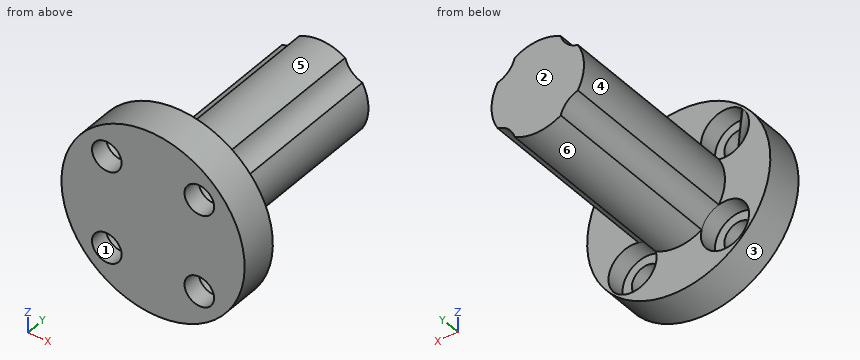
```python
from build123d import *
from build123d.topology import SkipClean

# Parameters (mm, degrees)
SKETCH1_R           = 9.9
BOSS_EXTRUDE1_DEPTH = 4
SKETCH2_R           = 5
BOSS_EXTRUDE2_DEPTH = 20
CUT_EXTRUDE1_REACH  = 26.414
SKETCH3_R           = 1.6
CUT_EXTRUDE2_REACH  = 26.414
SKETCH3_3_R         = 2.6
SKETCH3_3_R_2       = 1.6
SKETCH3_4_R         = 2.6
SKETCH3_4_R_2       = 1.6
CUT_EXTRUDE3_DEPTH  = 2


with BuildPart() as part:
    # Sketch1 → Boss-Extrude1 (new body)
    with BuildSketch(Plane(origin=(0, 0, 0), x_dir=(1, 0, 0), z_dir=(0, 1, 0))):
        with Locations(Location((0, 0, 0), (0, 0, 270))):
            Circle(SKETCH1_R)
    extrude(amount=BOSS_EXTRUDE1_DEPTH)

    # Sketch2 → Boss-Extrude2 (add)
    with BuildSketch(Plane(origin=(0, 4, 0), x_dir=(1, 0, 0), z_dir=(0, 1, 0))):
        with Locations(Location((0, 0, 0), (0, 0, 270))):
            Circle(SKETCH2_R)
    extrude(amount=BOSS_EXTRUDE2_DEPTH)

    # Sketch3 → Cut-Extrude1 (cut, up to next)
    with BuildSketch(Plane(origin=(0, 4, 0), x_dir=(1, 0, 0), z_dir=(0, 1, 0)), mode=Mode.PRIVATE) as cut_extrude1_sk1:
        with Locations(Location((5, 5, 0), (0, 0, 270))):
            Circle(SKETCH3_R)
    cut_extrude1_tool1 = extrude(cut_extrude1_sk1.sketch, amount=-CUT_EXTRUDE1_REACH, mode=Mode.PRIVATE) & part.part
    # Sketch3 → Cut-Extrude1 (cut, up to next)
    with BuildSketch(Plane(origin=(0, 4, 0), x_dir=(1, 0, 0), z_dir=(0, 1, 0)), mode=Mode.PRIVATE) as cut_extrude1_sk2:
        with Locations(Location((5, -5, 0), (0, 0, 270))):
            Circle(SKETCH3_R)
    cut_extrude1_tool2 = extrude(cut_extrude1_sk2.sketch, amount=-CUT_EXTRUDE1_REACH, mode=Mode.PRIVATE) & part.part
    # Sketch3 → Cut-Extrude1 (cut, up to next)
    with BuildSketch(Plane(origin=(0, 4, 0), x_dir=(1, 0, 0), z_dir=(0, 1, 0)), mode=Mode.PRIVATE) as cut_extrude1_sk3:
        with Locations(Location((-5, -5, 0), (0, 0, 270))):
            Circle(SKETCH3_R)
    cut_extrude1_tool3 = extrude(cut_extrude1_sk3.sketch, amount=-CUT_EXTRUDE1_REACH, mode=Mode.PRIVATE) & part.part
    # Sketch3 → Cut-Extrude1 (cut, up to next)
    with BuildSketch(Plane(origin=(0, 4, 0), x_dir=(1, 0, 0), z_dir=(0, 1, 0)), mode=Mode.PRIVATE) as cut_extrude1_sk4:
        with Locations(Location((-5, 5, 0), (0, 0, 270))):
            Circle(SKETCH3_R)
    cut_extrude1_tool4 = extrude(cut_extrude1_sk4.sketch, amount=-CUT_EXTRUDE1_REACH, mode=Mode.PRIVATE) & part.part
    add(cut_extrude1_tool1.solids().sort_by_distance((5, 4, -5))[0], mode=Mode.SUBTRACT)
    add(cut_extrude1_tool2.solids().sort_by_distance((5, 4, 5))[0], mode=Mode.SUBTRACT)
    add(cut_extrude1_tool3.solids().sort_by_distance((-5, 4, 5))[0], mode=Mode.SUBTRACT)
    add(cut_extrude1_tool4.solids().sort_by_distance((-5, 4, -5))[0], mode=Mode.SUBTRACT)

    # Sketch3_3 → Cut-Extrude2 (cut, up to next)
    with BuildSketch(Plane(origin=(0, 4, 0), x_dir=(1, 0, 0), z_dir=(0, 1, 0)), mode=Mode.PRIVATE) as cut_extrude2_sk1:
        with Locations((5, 5)):
            Circle(SKETCH3_3_R)
        with Locations(Location((5, 5, 0), (0, 0, 270))):
            Circle(SKETCH3_3_R_2, mode=Mode.SUBTRACT)
    cut_extrude2_tool1 = extrude(cut_extrude2_sk1.sketch, amount=CUT_EXTRUDE2_REACH, mode=Mode.PRIVATE) & part.part
    # Sketch3_3 → Cut-Extrude2 (cut, up to next)
    with BuildSketch(Plane(origin=(0, 4, 0), x_dir=(1, 0, 0), z_dir=(0, 1, 0)), mode=Mode.PRIVATE) as cut_extrude2_sk2:
        with Locations((-5, 5)):
            Circle(SKETCH3_3_R)
        with Locations(Location((-5, 5, 0), (0, 0, 270))):
            Circle(SKETCH3_3_R_2, mode=Mode.SUBTRACT)
    cut_extrude2_tool2 = extrude(cut_extrude2_sk2.sketch, amount=CUT_EXTRUDE2_REACH, mode=Mode.PRIVATE) & part.part
    # Sketch3_3 → Cut-Extrude2 (cut, up to next)
    with BuildSketch(Plane(origin=(0, 4, 0), x_dir=(1, 0, 0), z_dir=(0, 1, 0)), mode=Mode.PRIVATE) as cut_extrude2_sk3:
        with Locations((-5, -5)):
            Circle(SKETCH3_3_R)
        with Locations(Location((-5, -5, 0), (0, 0, 270))):
            Circle(SKETCH3_3_R_2, mode=Mode.SUBTRACT)
    cut_extrude2_tool3 = extrude(cut_extrude2_sk3.sketch, amount=CUT_EXTRUDE2_REACH, mode=Mode.PRIVATE) & part.part
    # Sketch3_3 → Cut-Extrude2 (cut, up to next)
    with BuildSketch(Plane(origin=(0, 4, 0), x_dir=(1, 0, 0), z_dir=(0, 1, 0)), mode=Mode.PRIVATE) as cut_extrude2_sk4:
        with Locations((5, -5)):
            Circle(SKETCH3_3_R)
        with Locations(Location((5, -5, 0), (0, 0, 270))):
            Circle(SKETCH3_3_R_2, mode=Mode.SUBTRACT)
    cut_extrude2_tool4 = extrude(cut_extrude2_sk4.sketch, amount=CUT_EXTRUDE2_REACH, mode=Mode.PRIVATE) & part.part
    add(cut_extrude2_tool1.solids().sort_by_distance((2.473539, 4, -5))[0], mode=Mode.SUBTRACT)
    add(cut_extrude2_tool2.solids().sort_by_distance((-7.526461, 4, -5))[0], mode=Mode.SUBTRACT)
    add(cut_extrude2_tool3.solids().sort_by_distance((-7.526461, 4, 5))[0], mode=Mode.SUBTRACT)
    add(cut_extrude2_tool4.solids().sort_by_distance((2.473539, 4, 5))[0], mode=Mode.SUBTRACT)

    # Sketch3_4 → Cut-Extrude3 (cut)
    # profile 1 of 4: a face of its own
    with SkipClean():  # the faces are left unmerged after this step: merging them gives an invalid solid
        with BuildSketch(Plane(origin=(0, 4, 0), x_dir=(1, 0, 0), z_dir=(0, 1, 0))):
            with Locations(Location((5, 5, 0), (0, 0, 194.741200994))):
                Circle(SKETCH3_4_R)
            with Locations(Location((5, 5, 0), (0, 0, 270))):
                Circle(SKETCH3_4_R_2, mode=Mode.SUBTRACT)
        # profile 2 of 4: a face of its own
        with BuildSketch(Plane(origin=(0, 4, 0), x_dir=(1, 0, 0), z_dir=(0, 1, 0))):
            with Locations(Location((-5, 5, 0), (0, 0, 345.258799006))):
                Circle(SKETCH3_4_R)
            with Locations(Location((-5, 5, 0), (0, 0, 270))):
                Circle(SKETCH3_4_R_2, mode=Mode.SUBTRACT)
        # profile 3 of 4: a face of its own
        with BuildSketch(Plane(origin=(0, 4, 0), x_dir=(1, 0, 0), z_dir=(0, 1, 0))):
            with Locations(Location((-5, -5, 0), (0, 0, 75.258799006))):
                Circle(SKETCH3_4_R)
            with Locations(Location((-5, -5, 0), (0, 0, 270))):
                Circle(SKETCH3_4_R_2, mode=Mode.SUBTRACT)
        # profile 4 of 4: a face of its own
        with BuildSketch(Plane(origin=(0, 4, 0), x_dir=(1, 0, 0), z_dir=(0, 1, 0))):
            with Locations(Location((5, -5, 0), (0, 0, 104.741200994))):
                Circle(SKETCH3_4_R)
            with Locations(Location((5, -5, 0), (0, 0, 270))):
                Circle(SKETCH3_4_R_2, mode=Mode.SUBTRACT)
        extrude(amount=-CUT_EXTRUDE3_DEPTH, mode=Mode.SUBTRACT)


solid = part.part
```
Geometry: final body of the model. Coordinates: model frame, mm. Face numbers are marked on the shaded views. A direction names the side the tool comes from. Coordinates: 2 decimals unless noted, no trailing zeros. Order: outer loops, then holes, each group sorted by start corner. A loop starts at its lowest first (then second) coordinate and runs counter-clockwise, first axis right, second up.
Item 1: Draft query along X for the marked faces 1, 2 and 3. Return one class per face: released by +X, released by -X, zero draft, split by the parting line, or undercut.
Answer:
face 1: undercut
face 2: zero draft
face 3: split by the parting line
Item 2: Section query C-C (x = 0). Output: boundary loops of the cut face in (y, z), then the cut area to 3 significant figures.
Answer:
outline: (0, -9.9) - (4, -9.9) - (4, -5) - (24, -5) - (24, 5) - (4, 5) - (4, 9.9) - (0, 9.9) - close
area: 279 mm2
Item 3: Section query A-A (x = 5.5). Output: boundary loops of the cut face in (y, z).
Answer:
outline: (0, -8.23) - (4, -8.23) - (4, -7.55) - (2, -7.55) - (2, -6.52) - (0, -6.52) - close; (0, -3.48) - (2, -3.48) - (2, -2.45) - (4, -2.45) - (4, 2.45) - (2, 2.45) - (2, 3.48) - (0, 3.48) - close; (0, 6.52) - (2, 6.52) - (2, 7.55) - (4, 7.55) - (4, 8.23) - (0, 8.23) - close
Item 4: Access query for the marked faces 4, 5 and 6. Directions: +Z, -Z, +X, -X, +Y, -Y. A direction counts if a zero-diameter tool reaches every point of the face in a straight line with its end or side. Return the directions, or none.
Answer:
face 4: -X, +Y
face 5: +Z, +Y
face 6: -Z, +Y
Item 5: Section query D-D (z = -7). Output: boundary loops of the cut face in (x, y), then the cut area to 3 significant figures.
Answer:
outline: (-7, 0) - (7, 0) - (7, 4) - (6.66, 4) - (6.66, 2) - (3.34, 2) - (3.34, 4) - (-3.34, 4) - (-3.34, 2) - (-6.66, 2) - (-6.66, 4) - (-7, 4) - close
area: 42.7 mm2
Item 6: Section query B-B (z = 0). Output: boundary loops of the cut face in (x, y).
Answer:
outline: (-9.9, 0) - (9.9, 0) - (9.9, 4) - (5, 4) - (5, 24) - (-5, 24) - (-5, 4) - (-9.9, 4) - close
Item 7: Contact query for flat-ended pins moving along their axis: P1, Ø7, axis at x = -5, z = -5, coming from the -Y side; P2, Ø2.5, axis at x = -6, z = 4, coming from the +Y side; P3, Ø5, axis at x = -5, z = -5, coming from the +Y side; P4, Ø1, axis at x = -1, y = 16, coming from the -Z side. Output: stop coordinate, or through.
Answer:
P1: stops at y = 0
P2: stops at y = 4
P3: stops at y = 2
P4: stops at z = -4.97
